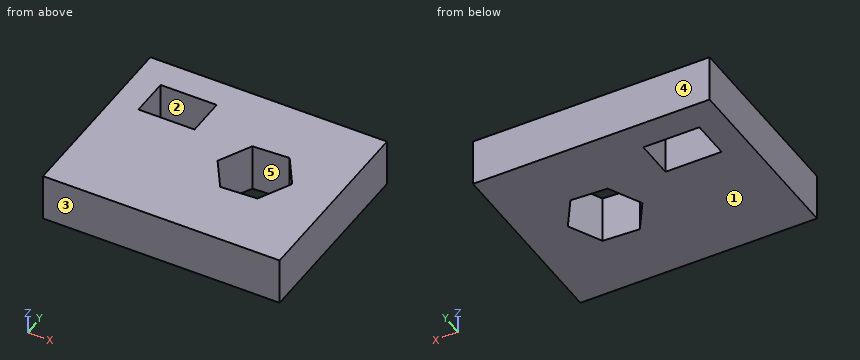
from build123d import *

# Parameters (mm, degrees)
SKETCH_W   = 50
SKETCH_H   = 40
SKETCH_W_2 = 11.856175
SKETCH_H_2 = 8.260444
PAD_DEPTH  = 10


with BuildPart() as part:
    # Sketch → Pad (new body)
    with BuildSketch(Plane.XY):
        with Locations((25, 20)):
            Rectangle(SKETCH_W, SKETCH_H)
        with Locations((11.564625, 29.737606)):
            Rectangle(SKETCH_W_2, SKETCH_H_2, mode=Mode.SUBTRACT)
        Polygon((37.512146, 13.751215), (40.977424, 20.577169), (36.798614, 26.991165), (29.154526, 26.579207), (25.689248, 19.753253), (29.868058, 13.339257), align=None, mode=Mode.SUBTRACT)
    extrude(amount=PAD_DEPTH)


solid = part.part
The model under review builds one solid part; all positions refer to its coordinate system, in mm. Face numbers are marked on the shaded views. A direction names the side the tool comes from. Coordinates: 2 decimals unless noted, no trailing zeros. Write each loop counter-clockwise with the first axis right and the second up, starting at its lowest first coordinate (ties: lowest second). Pieces come first, ordered by that corner, then holes. Notation, with made-up numbers: (85.5, -12) - (140.5, -12) arc R29 cw to (140.5, 18) - close; hole circle Ø11 at (1.5, -10). An arc over 180 degrees is marked (long way). Answer as a JSON object with one key per item and string values. Group by question number.
1. Add section C-C (z = 5.5). Give the boundary of the cut face in (x, y).
2. Mouldability with a two-part tool opening along Y and no side actions: class the marked faces 1, 2 and 3 as pulls with the +Y half, pulls with the -Y half, needs draft (parallel to the pull), parting line crosses it, or undercut.
3. Add section A-A (x = 12). Give the boundary of the cut face in (y, z), plus the area to 3 significant figures.
4. Machinability: for the marked faces 4 and 5, which of the approach directions +Z, -Z, +X, -X, +Y, -Y give a long, thin tool a straight path to every point of the face, cutting with its end or side? Answer none if there is none.
5. Clearance check with a flat-ended pin moving along its axis: pin 1 Ø5 at (x, z) = (6, 4.5) entering from -Y. State where the tip first meets the part, or that it passes through.
6. Add section B-B (y = 29). Give the boundary of the cut face in (x, z), plus the area to 3 significant figures.
7. To check wall thickness, follow probe 1 along Y at (x, z) = (10.5, 1.75); probe 2 along X at (y, z) = (30, 8.75); probe 3 along Y at (x, z) = (33.5, 8.25) (3 decimals). State the ranges of each line that lie inside material, in increasing order.
Findings:
{
 "1": {"outline": "(0, 0) - (50, 0) - (50, 40) - (0, 40) - close; hole (5.64, 25.61) - (17.49, 25.61) - (17.49, 33.87) - (5.64, 33.87) - close; hole (25.69, 19.75) - (29.87, 13.34) - (37.51, 13.75) - (40.98, 20.58) - (36.8, 26.99) - (29.15, 26.58) - close"},
 "2": {"face 1": "needs draft", "face 2": "undercut", "face 3": "pulls with the -Y half"},
 "3": {"outline": "(0, 0) - (25.61, 0) - (25.61, 10) - (0, 10) - close; (33.87, 0) - (40, 0) - (40, 10) - (33.87, 10) - close", "area": "317 mm²"},
 "4": {"face 4": "+Z, -Z, +X, -X, +Y", "face 5": "+Z, -Z"},
 "5": {"pin 1": "y = 0"},
 "6": {"outline": "(0, 0) - (5.64, 0) - (5.64, 10) - (0, 10) - close; (17.49, 0) - (50, 0) - (50, 10) - (17.49, 10) - close", "area": "381 mm²"},
 "7": {"probe 1": "0 to 25.61, 33.87 to 40", "probe 2": "0 to 5.64, 17.49 to 50", "probe 3": "0 to 13.535, 26.813 to 40"}
}
